```python
from build123d import *

# Parameters (mm, degrees)
SKETCH1_W            = 51.054
SKETCH1_H            = 50.8
BOSS_EXTRUDE1_DEPTH  = 2.3622
SKETCH5_R            = 2.921
BOSS_EXTRUDE3_DEPTH  = 0.254
SKETCH2_R            = 1.524
CUT_EXTRUDE1_DEPTH   = 73.060605776
LPATTERN1_COUNT      = 2
LPATTERN1_PITCH      = 43.18
LPATTERN1_COUNT_DIR2 = 2
LPATTERN1_PITCH_DIR2 = 43.18
FILLET1_R            = 2.54
SKETCH3_R            = 1.27
CUT_EXTRUDE2_DEPTH   = 73.060605776
SKETCH6_W            = 1.524
SKETCH6_H            = 1.524
BOSS_EXTRUDE4_DEPTH  = 0.254
LPATTERN2_COUNT      = 7
LPATTERN2_PITCH      = 2.54


with BuildPart() as part:
    # Sketch1 → Boss-Extrude1 (new body)
    with BuildSketch(Plane(origin=(0, 0, 0), x_dir=(1, 0, 0), z_dir=(0, 1, 0))):
        with Locations((25.527, 25.4)):
            Rectangle(SKETCH1_W, SKETCH1_H)
    extrude(amount=BOSS_EXTRUDE1_DEPTH)

    # Sketch5 → Boss-Extrude3 (add)
    with BuildSketch(Plane(origin=(0, 2.3622, 0), x_dir=(1, 0, 0), z_dir=(0, 1, 0))):
        with Locations(Location((3.81, 3.81, 0), (0, 0, 90))):
            Circle(SKETCH5_R)
    boss_extrude3 = extrude(amount=BOSS_EXTRUDE3_DEPTH)

    # Sketch2 → Cut-Extrude1 (cut, symmetric)
    with BuildSketch(Plane(origin=(0, 2.3622, 0), x_dir=(1, 0, 0), z_dir=(0, 1, 0))):
        with Locations(Location((3.81, 3.81, 0), (0, 0, 270))):
            Circle(SKETCH2_R)
    cut_extrude1 = extrude(amount=CUT_EXTRUDE1_DEPTH, both=True, mode=Mode.SUBTRACT)

    # LPattern1: Boss-Extrude3, Cut-Extrude1 2 × 2
    with Locations(*[(j * LPATTERN1_PITCH_DIR2, 0, -i * LPATTERN1_PITCH) for i in range(LPATTERN1_COUNT) for j in range(LPATTERN1_COUNT_DIR2) if (i, j) != (0, 0)]):
        add(boss_extrude3)
        add(cut_extrude1, mode=Mode.SUBTRACT)

    # Fillet1
    fillet1_edges = [part.edges().sort_by_distance(p)[0] for p in [
        (0, 1.1811, -50.8),
        (51.054, 1.1811, -50.8),
        (51.054, 1.1811, 0),
        (0, 1.1811, 0),
    ]]
    fillet(fillet1_edges, radius=FILLET1_R)

    # Sketch3 → Cut-Extrude2 (cut, through all)
    with BuildSketch(Plane(origin=(0, 2.3622, 0), x_dir=(1, 0, 0), z_dir=(0, 1, 0))):
        with Locations(Location((25.4, 4.443185344, 0), (0, 0, 270))):
            Circle(SKETCH3_R)
    extrude(amount=-CUT_EXTRUDE2_DEPTH, mode=Mode.SUBTRACT)

    # Sketch6 → Boss-Extrude4 (add)
    with BuildSketch(Plane(origin=(0, 2.3622, 0), x_dir=(1, 0, 0), z_dir=(0, 1, 0))):
        with Locations((50.165, 35.56)):
            Rectangle(SKETCH6_W, SKETCH6_H)
    boss_extrude4 = extrude(amount=BOSS_EXTRUDE4_DEPTH)

    # LPattern2: Boss-Extrude4 ×7
    with Locations(*[(0, 0, i * LPATTERN2_PITCH) for i in range(1, LPATTERN2_COUNT)]):
        add(boss_extrude4)


solid = part.part
```
Can you work these out from the model? Positions are in its coordinate system, mm. Coordinates: 2 decimals unless noted, no trailing zeros. Order: outer loops, then holes, each group sorted by start corner. A loop starts at its lowest first (then second) coordinate and runs counter-clockwise, first axis right, second up.
1. Thinking about a two-plate mould opening in Z: for faces 1 (the face through (4.84, 1.326, -4.933)), 2 (the face through (48.2, 2.616, -48.2)), 3 (the face through (4.268, 1.326, -45.536)), 4 (the face through (50.29, 1.198, -0.724)), which applies, +Z half, -Z half, draft (parallel to the pull), parting line (faces both ways), or undercut?
2. I need wall thicknesses on line 1 (X direction, y = 1.3, z = -46.99); line 2 (X direction, y = 1.45, z = -5); line 3 (X direction, y = 0.8, z = -3.81). Which ranges of each line are inside material? Lowest first, please.
3. If we section it at C-C (y = 1.05): Please give me the cut outline in (x, z).
4. If we section it at D-D (z = -3.81): Please give me the cut outline in (x, y).
5. If we section it at B-B (x = 3.81): Please give me the cut outline in (y, z).
6. If we section it at A-A (x = 25.4): Please give me the cut outline in (y, z), then the cut area to 3 significant figures.
Entries:
1. face 1: undercut
1. face 2: draft
1. face 3: undercut
1. face 4: +Z half
2. line 1: x = 0 to 2.29, 5.33 to 45.47, 48.51 to 51.05
2. line 2: x = 0 to 2.86, 4.76 to 24.26, 26.54 to 46.04, 47.94 to 51.05
2. line 3: x = 0 to 2.29, 5.33 to 24.3, 26.5 to 45.47, 48.51 to 51.05
3. outline: (0, -48.26) arc R2.54 ccw to (2.54, -50.8) - (48.51, -50.8) arc R2.54 ccw to (51.05, -48.26) - (51.05, -2.54) arc R2.54 ccw to (48.51, 0) - (2.54, 0) arc R2.54 ccw to (0, -2.54) - close; hole circle Ø3.05 at (3.81, -46.99); hole circle Ø3.05 at (3.81, -3.81); hole circle Ø2.54 at (25.4, -4.44); hole circle Ø3.05 at (46.99, -46.99); hole circle Ø3.05 at (46.99, -3.81)
4. outline: (0, 0) - (2.29, 0) - (2.29, 2.62) - (0.89, 2.62) - (0.89, 2.36) - (0, 2.36) - close; (5.33, 0) - (24.3, 0) - (24.3, 2.36) - (6.73, 2.36) - (6.73, 2.62) - (5.33, 2.62) - close; (26.5, 0) - (45.47, 0) - (45.47, 2.62) - (44.07, 2.62) - (44.07, 2.36) - (26.5, 2.36) - close; (48.51, 0) - (51.05, 0) - (51.05, 2.36) - (49.91, 2.36) - (49.91, 2.62) - (48.51, 2.62) - close
5. outline: (0, -50.8) - (2.36, -50.8) - (2.36, -49.91) - (2.62, -49.91) - (2.62, -48.51) - (0, -48.51) - close; (0, -45.47) - (2.62, -45.47) - (2.62, -44.07) - (2.36, -44.07) - (2.36, -6.73) - (2.62, -6.73) - (2.62, -5.33) - (0, -5.33) - close; (0, -2.29) - (2.62, -2.29) - (2.62, -0.89) - (2.36, -0.89) - (2.36, 0) - (0, 0) - close
6. outline: (0, -50.8) - (2.36, -50.8) - (2.36, -5.71) - (0, -5.71) - close; (0, -3.17) - (2.36, -3.17) - (2.36, 0) - (0, 0) - close
6. area: 114 mm2
